CAD build for the part. Positions are in the model's coordinates, mm. Round coordinates to 2 decimals unless told otherwise and drop trailing zeros. Write each loop counter-clockwise with the first axis right and the second up, starting at its lowest first coordinate (ties: lowest second). Pieces come first, ordered by that corner, then holes. Notation, with made-up numbers: (-22, 53.25) -> (-1, 53.25) arc R23 ccw to (-1, 72.25) -> close; hole circle Ø4 at (36.5, 7). An arc over 180 degrees is marked (long way). Put each result on its own line as item: value. Start each with the question number.
1. Flat gauge pins, fed straight in: P1, Ø6, axis at y = 14.5, z = 18.5, coming from the -X side; P2, Ø8, axis at y = 12, z = -1, coming from the +X side; P3, Ø4, axis at x = -74.5, z = 5.5, coming from the -Y side. Where does each tip first touch, or does it go through?
2. Saw through at B-B on z = -16. List the corners of the cut face in (x, y).
3. Saw through at A-A on y = 3.75. List the corners of the cut face in (x, z), and give its area (3 significant figures).
4. Saw through at D-D on x = -32. List the corners of the cut face in (y, z), and give its area (3 significant figures).
5. Saw through at C-C on y = 21.5. List the corners of the cut face in (x, z).
6. Drill centre lines: line 1 (X direction, y = 16.25, z = 7.5); line 2 (Z direction, x = -74.5, y = 11); line 3 (X direction, y = 6, z = -13). Where is each one in solid material? Low to high. Write a range as from..to.
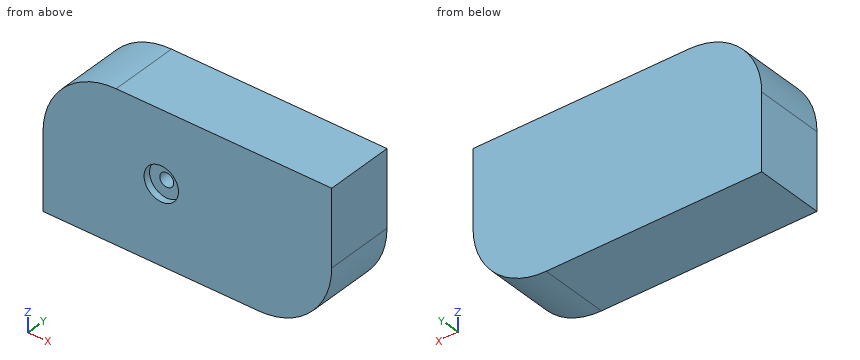
from build123d import *

# Parameters (mm, degrees)
F0_W           = 106.4566392452
F0_H           = 55.0185795873
F1_DEPTH       = 25.4
F2_R           = 26.9812507731
F3_D           = 5.08
F3_DEPTH       = 13.6525
F3_CBORE_D     = 12.7
F3_CBORE_DEPTH = 2.5146
F3_TIP         = 1.5261859723


with BuildPart() as f1:
    # F0 (on Front) → F1 (new body)
    with BuildSketch(Plane.XZ):
        with Locations((-65.4772659764, 6.4995298162)):
            Rectangle(F0_W, F0_H)
    extrude(amount=-F1_DEPTH)

    # F2
    f2_edges = [f1.edges().sort_by_distance(p)[0] for p in [
        (-12.248946, 12.7, -21.00976),
        (-118.705586, 12.7, 34.00882),
    ]]
    fillet(f2_edges, radius=F2_R)

    # F3
    with Locations(Plane.XZ):
        with Locations((-75.099773705, 7.8630894423)):
            CounterBoreHole(F3_D / 2, F3_CBORE_D / 2, F3_CBORE_DEPTH, depth=F3_DEPTH)
            with Locations((0, 0, -(F3_DEPTH + F3_TIP / 2))):  # 118° drill point
                Cone(0, F3_D / 2, F3_TIP, mode=Mode.SUBTRACT)


solid = f1.part
Return value:
1. P1: stops at x = -117.34
1. P2: stops at x = -12.41
1. P3: stops at y = 2.51
2. outline: (-118.71, 0) -> (-23.57, 0) -> (-23.57, 25.4) -> (-118.71, 25.4) -> close
3. outline: (-118.71, -21.01) -> (-39.23, -21.01) arc R26.98 ccw to (-12.25, 5.97) -> (-12.25, 34.01) -> (-91.72, 34.01) arc R26.98 ccw to (-118.71, 7.03) -> close; hole circle Ø5.08 at (-75.1, 7.86)
3. area: 5,520 mm^2
4. outline: (0, -20.02) -> (25.4, -20.02) -> (25.4, 34.01) -> (0, 34.01) -> close
4. area: 1,370 mm^2
5. outline: (-118.71, -21.01) -> (-39.23, -21.01) arc R26.98 ccw to (-12.25, 5.97) -> (-12.25, 34.01) -> (-91.72, 34.01) arc R26.98 ccw to (-118.71, 7.03) -> close
6. line 1: x = -118.7..-12.25
6. line 2: z = -21.01..5.39, 10.33..34.01
6. line 3: x = -118.71..-20.05
